from build123d import *

# Parameters (mm, degrees)
F1_DEPTH = 50
F4_DEPTH = 5
F6_DEPTH = 25
F8_D     = 3.3
F8_DEPTH = 13.5
F8_TIP   = 0.9914200214


with BuildPart() as f1:
    # F0 (on Front) → F1 (new body)
    with BuildSketch(Plane.XZ):
        Polygon((0, 0), (21, 0), (21, 1), (12, 1), (12, 28), (0, 28), align=None)
    extrude(amount=-F1_DEPTH)

    # F2: F1 across plane


with BuildPart() as f1_1:
    add(f1.part)
    add(f1.part.mirror(Plane.YZ))

    # F3 (on Right) → F4 (join, symmetric)
    with BuildSketch(Plane.YZ):
        Polygon((0, 18), (-1.5, 18), (-11.5, 8), (0, 8), align=None)
    extrude(amount=F4_DEPTH, both=True)

    # F5 (on face) → F6 (intersect)
    with BuildSketch(Plane(origin=(0, 0, 0), x_dir=(1, 0, 0), z_dir=(0, 0, -1))):
        Polygon((-12, 0), (-12, -50), (12, -50), (12, 0), (12, 11.5), (-12, 11.5), align=None)
    extrude(amount=-F6_DEPTH, mode=Mode.INTERSECT)

    # F8
    with Locations(Plane(origin=(0, 0, 0), x_dir=(1, 0, 0), z_dir=(0, 0, -1))):
        with Locations((7, -20), (7, -40), (-7, -40), (-7, -20)):
            Hole(F8_D / 2, depth=F8_DEPTH)
            with Locations((0, 0, -(F8_DEPTH + F8_TIP / 2))):  # 118° drill point
                Cone(0, F8_D / 2, F8_TIP, mode=Mode.SUBTRACT)


solid = f1_1.part
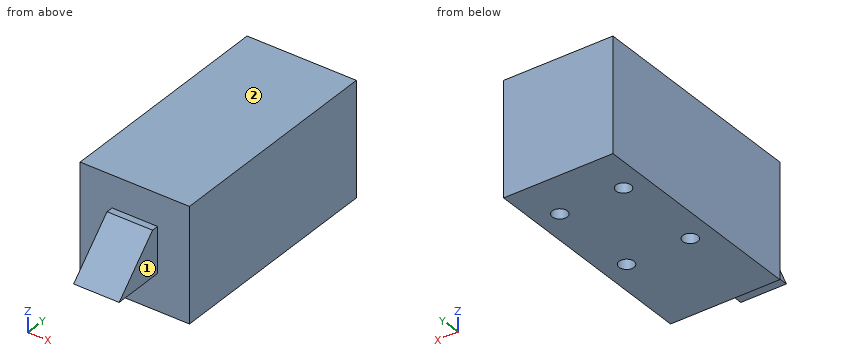
Part model, mm, in its own coordinate system. Face numbers are marked on the shaded views. A direction names the side the tool comes from. Coordinates: 2 decimals unless noted, no trailing zeros. Loops run counter-clockwise (first coordinate to the right, second up) from the corner with the lowest first, then second, coordinate; pieces in that order, holes last. Notation, with made-up numbers: M 82.5,-6 L 130.5,-6 A8 ccw 130.5,1 Z; hole C 65.25,-3.5 d3. An arc over 180 degrees is marked long. Use a Markdown table: item, result. Add a question column.
Q1. Cut at A-A (z = 11.5). Write the cut outline in (x, y).
Q2. Cut at C-C (z = 22.25). Write the cut outline in (x, y), and give its area (3 significant figures).
Q3. Pin check, flat tips, straight feed: P1, Ø7, axis at x = -1, z = 16, coming from the -Y side; P2, Ø8, axis at x = -1, y = -6.5, coming from the -Z side; P3, Ø5, axis at y = -8, z = 13, coming from the -X side. Stop position of each tip, or through.
Q4. Probe L1, parallel to Y at x = 7, z = 5; L2, parallel to X at y = 20, z = 7; L3, parallel to X at y = 21, z = 7.25. List the from-to ranges inside material, lowest first.
Q5. Cut at D-D (x = 10.75). Write the cut outline in (y, z).
Q6. Cut at B-B (x = 2.75). Write the cut outline in (y, z).
Q7. Which spindle directions (+Z, -Z, +X, -X, +Y, -Y) get a long thin tool onto all of the face, cutting with end or side? Do the marked faces 1 and 2. Say none if no direction does.
Worked out:
| question | item | result |
|---|---|---|
| 1 | outline | M -12,0 L -5,0 L -5,-8 L 5,-8 L 5,0 L 12,0 L 12,50 L -12,50 Z; hole C -7,20 d3.3; hole C -7,40 d3.3; hole C 7,20 d3.3; hole C 7,40 d3.3 |
| 2 | outline | M -12,0 L 12,0 L 12,50 L -12,50 Z |
| 2 | area | 1,200 mm2 |
| 3 | P1 | stops at y = -7 |
| 3 | P2 | stops at z = 8 |
| 3 | P3 | stops at x = -5 |
| 4 | L1 | y = 0 to 18.35, 21.65 to 38.35, 41.65 to 50 |
| 4 | L2 | x = -12 to -8.65, -5.35 to 5.35, 8.65 to 12 |
| 4 | L3 | x = -12 to -8.31, -5.69 to 5.69, 8.31 to 12 |
| 5 | outline | M 0,0 L 50,0 L 50,25 L 0,25 Z |
| 6 | outline | M -11.5,8 L 0,8 L 0,0 L 50,0 L 50,25 L 0,25 L 0,18 L -1.5,18 Z |
| 7 | face 1 | +Z, -Z, +X, -Y |
| 7 | face 2 | +Z, +X, -X, +Y, -Y |
